```python
from build123d import *

# Parameters (mm, degrees)
F1_DEPTH = 25


with BuildPart() as f1:
    # F0 (on Front) → F1 (new body)
    with BuildSketch(Plane.XZ):
        with BuildLine():
            ThreePointArc((-42.592177, 32.152407), (-46.127711, 30.687941), (-47.592177, 27.152407))
            Line((-47.592177, 27.152407), (-47.592177, -17.847593))
            ThreePointArc((-47.592177, -17.847593), (-46.127711, -21.383127), (-42.592177, -22.847593))
            Line((-42.592177, -22.847593), (52.407823, -22.847593))
            ThreePointArc((52.407823, -22.847593), (67.407823, -7.847593), (52.407823, 7.152407))
            Line((52.407823, 7.152407), (12.407823, 7.152407))
            ThreePointArc((12.407823, 7.152407), (5.336755, 10.081339), (2.407823, 17.152407))
            Line((2.407823, 17.152407), (2.407823, 32.152407))
            Line((2.407823, 32.152407), (-7.592177, 32.152407))
            ThreePointArc((-7.592177, 32.152407), (-22.592177, 17.152407), (-37.592177, 32.152407))
            Line((-37.592177, 32.152407), (-42.592177, 32.152407))
        make_face()
    extrude(amount=F1_DEPTH)


solid = f1.part
```
Could you check a few things on this model? Use its own coordinates, in mm. A direction names the side the tool comes from. Coordinates: 2 decimals unless noted, no trailing zeros. Write each loop counter-clockwise with the first axis right and the second up, starting at its lowest first coordinate (ties: lowest second). Pieces come first, ordered by that corner, then holes. Notation, with made-up numbers: (9.25, 5.25) -> (57.25, 5.25) arc R16 cw to (57.25, 21.25) -> close; hole circle Ø1 at (35.5, 1). An arc over 180 degrees is marked (long way). One line per question, with ' | ' between items. Start each with the question number.
1. For faces 1 (the face through (33, -12, 7.152)), 2 (the face through (-4, -25, -1)), which set-ups out of +Z, -Z, +X, -X, +Y, -Y let a thin tool reach every point of the face, with its end or its side?
2. If we section it at C-C (x = 35.5): Please give me the cut outline in (y, z), and give its area (3 significant figures).
3. If we section it at D-D (z = 14): Please give me the cut outline in (x, y).
4. If we section it at B-B (z = 23): Please give me the cut outline in (x, y), and give its area (3 significant figures).
5. If we section it at A-A (y = -17.25): Please give me the cut outline in (x, z), and give its area (3 significant figures).
6. Will these pins go through, and if not, where does the flat tip stop? P1, Ø8, axis at y = -16, z = -2.5, coming from the +X side; P2, Ø2, axis at x = 38.5, y = -15, coming from the +Z side.
7. Please list where these lines run through material, in increasing order: line 1 along Z through (x, y) = (22, -17.75); line 2 along X through (y, z) = (-15.5, 23.5); line 3 along X through (y, z) = (-17.5, 23).
Return value:
1) face 1: +Z, +X, +Y, -Y | face 2: +Z, -Z, +X, -X, -Y
2) outline: (-25, -22.85) -> (0, -22.85) -> (0, 7.15) -> (-25, 7.15) -> close | area: 750 mm²
3) outline: (-47.59, -25) -> (2.92, -25) -> (2.92, 0) -> (-47.59, 0) -> close
4) outline: (-47.59, -25) -> (-34.48, -25) -> (-34.48, 0) -> (-47.59, 0) -> close; (-10.71, -25) -> (2.41, -25) -> (2.41, 0) -> (-10.71, 0) -> close | area: 656 mm²
5) outline: (-47.59, -17.85) arc R5 ccw to (-42.59, -22.85) -> (52.41, -22.85) arc R15 ccw to (52.41, 7.15) -> (12.41, 7.15) arc R10 cw to (2.41, 17.15) -> (2.41, 32.15) -> (-7.59, 32.15) arc R15 cw to (-37.59, 32.15) -> (-42.59, 32.15) arc R5 ccw to (-47.59, 27.15) -> close | area: 4,260 mm²
6) P1: stops at x = 67.35 | P2: stops at z = 7.15
7) line 1: z = -22.85 to 7.15 | line 2: x = -47.59 to -34.85, -10.34 to 2.41 | line 3: x = -47.59 to -34.48, -10.71 to 2.41
